Geometry: see drawing. Coordinates: mm, zero at the bounding-box minimum. Coordinates: 2 decimals unless noted, no trailing zeros. Loops run counter-clockwise (first coordinate to the right, second up) from the corner with the lowest first, then second, coordinate; pieces in that order, holes last. Notation, with made-up numbers: (20.5, 35.25) - (63.5, 35.25) arc R28 ccw to (63.5, 66.25) - close; hole circle Ø4 at (55, 59). An arc over 180 degrees is marked (long way). Use a Markdown table: item, result. Add a question column.
1. Section query A-A on z = 25. Return the cut outline in (x, y).
2. Section query C-C on y = 4.5. Return the cut outline in (x, z), then the cut area to 3 significant figures.
3. Contact query for flat-ended pins moving along their axis: P1, Ø6.5, axis at x = 25, z = 25, coming from the +Y side; P2, Ø2, axis at x = 41.5, y = 12, coming from the -Z side (1 decimal); P3, Ø6, axis at x = 15.5, y = 10, coming from the -Z side; P4, Ø4, axis at y = 7.5, z = 43.5, coming from the -X side. Output: stop coordinate, or through.
4. Ray query, L1, parallel to Z at x = 25, y = 7; L2, parallel to X at y = 11, z = 22.5 (1 decimal); L3, parallel to Z at x = 28, y = 5.5 (1 decimal). Return the intervals inside material, ascending. Write a range as [from, to].
5. Section query D-D on z = 42. Return the cut outline in (x, y), then the cut area to 3 significant figures.
6. Draft query along Z for the marked faces 1, 2 and 3. Return one class per face: released by +Z, released by -Z, zero draft, split by the parting line, or undercut.
7. Section query B-B on x = 25. Return the cut outline in (y, z).
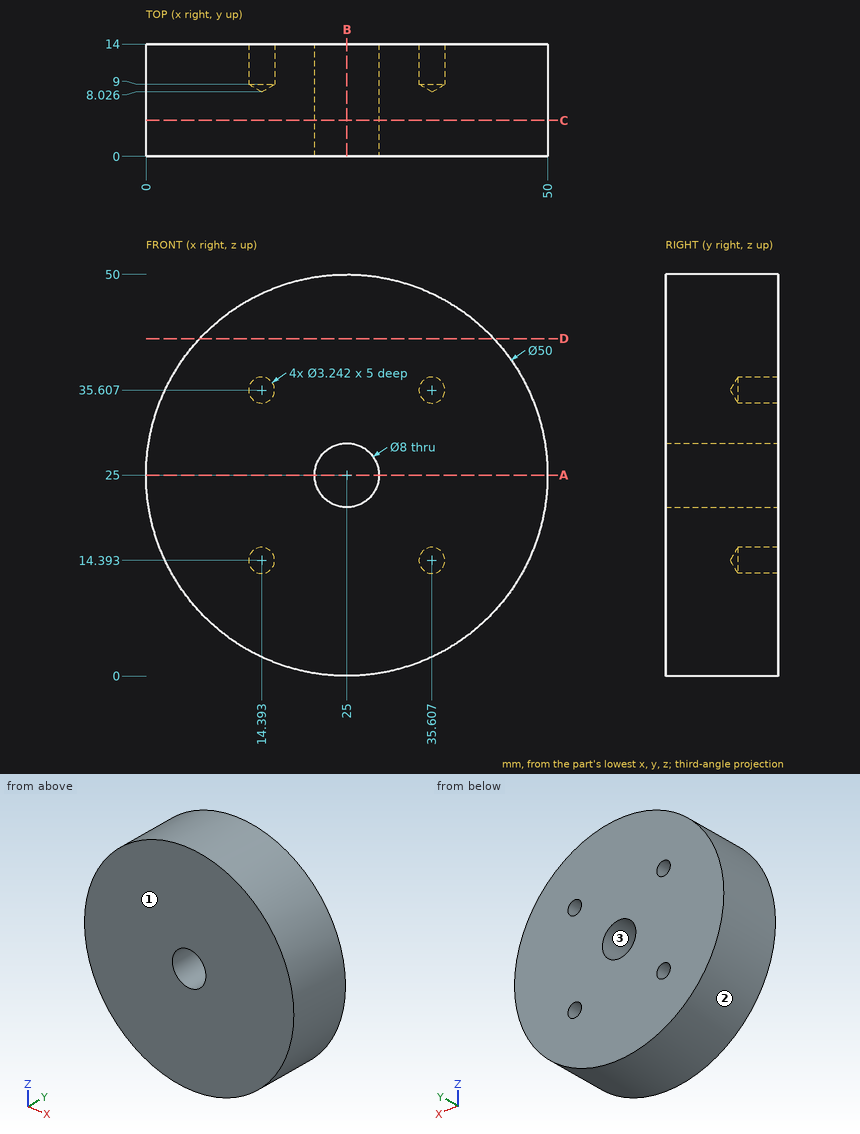
Resolved:
| question | item | result |
|---|---|---|
| 1 | outline | (0, 0) - (21, 0) - (21, 14) - (0, 14) - close; (29, 0) - (50, 0) - (50, 14) - (29, 14) - close |
| 2 | outline | circle Ø50 at (25, 25); hole circle Ø8 at (25, 25) |
| 2 | area | 1,910 mm² |
| 3 | P1 | through |
| 3 | P2 | z = 5.4 |
| 3 | P3 | z = 0.86 |
| 3 | P4 | x = 6.22 |
| 4 | L1 | [0, 21], [29, 50] |
| 4 | L2 | [0.1, 21.9], [28.1, 49.9] |
| 4 | L3 | [0.2, 22.4], [27.6, 49.8] |
| 5 | outline | (6.67, 0) - (43.33, 0) - (43.33, 14) - (6.67, 14) - close |
| 5 | area | 513 mm² |
| 6 | face 1 | zero draft |
| 6 | face 2 | split by the parting line |
| 6 | face 3 | undercut |
| 7 | outline | (0, 0) - (14, 0) - (14, 21) - (0, 21) - close; (0, 29) - (14, 29) - (14, 50) - (0, 50) - close |
